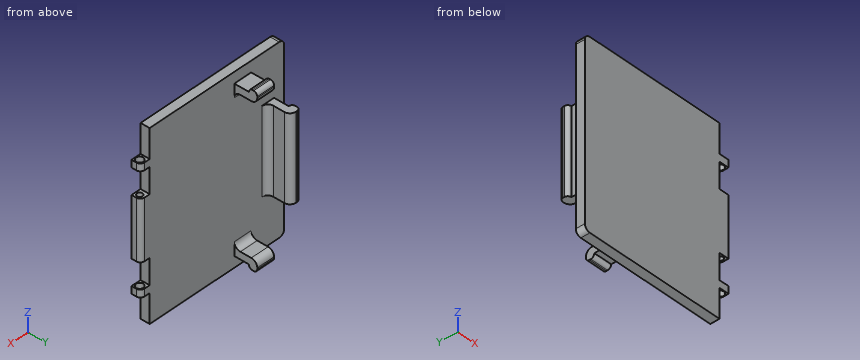
from build123d import *

# Parameters (mm, degrees)
EXTRUDE_START       = 0.25
EXTRUDE_BASE_DEPTH  = 3.75
FILLET1_R           = 1.75
SKETCH2_W           = 4
SKETCH2_H           = 10.5
SKETCH2_H_2         = 11.8971
CUT_EXTRUDE2_DEPTH  = 70.879033956
SKETCH4_R           = 1.5
CUT_EXTRUDE3_DEPTH  = 87.315736962
SKETCH6_W           = 3
SKETCH6_H           = 17.5
SKETCH6_W_2         = 7.5
SKETCH6_H_2         = 3
BOSS_EXTRUDE2_DEPTH = 9.5
SKETCH7_W           = 1.5
SKETCH7_H           = 3.5
BOSS_EXTRUDE3_DEPTH = 35
SKETCH8_W           = 1.5
SKETCH8_H           = 3.5
BOSS_EXTRUDE4_DEPTH = 7.5
SKETCH9_W           = 1.5
SKETCH9_H           = 3.5
BOSS_EXTRUDE5_DEPTH = 7.5
FILLET2_R           = 1.5
FILLET3_R           = 2.5
BOSS_EXTRUDE6_START = -24.5
SKETCH11_R          = 1.5
SKETCH11_R_2        = 1.125
BOSS_EXTRUDE6_DEPTH = 24.5


# Some blends are built 0.0001 mm under size
with BuildPart() as part:
    # Sketch1 → Extrude Base (new body)
    with BuildSketch(Plane.XZ.offset(10.085054916).offset(EXTRUDE_START)):
        with BuildLine():
            Line((56.857940404, 38.199863775), (56.857940404, -32.594336225))
            ThreePointArc((56.857940404, -32.594336225), (56.198930662, -34.185326483), (54.607940404, -34.844336225))
            Line((54.607940404, -34.844336225), (-4.892059596, -34.844336225))
            ThreePointArc((-4.892059596, -34.844336225), (-6.483049854, -34.185326483), (-7.142059596, -32.594336225))
            Line((-7.142059596, -32.594336225), (-7.142059596, 38.199863775))
            ThreePointArc((-7.142059596, 38.199863775), (-6.483049854, 39.790854032), (-4.892059596, 40.449863775))
            Line((-4.892059596, 40.449863775), (54.607940404, 40.449863775))
            ThreePointArc((54.607940404, 40.449863775), (56.198930662, 39.790854032), (56.857940404, 38.199863775))
        make_face()
    extrude(amount=EXTRUDE_BASE_DEPTH)

    # Fillet1
    # the kernel refuses this fillet: 1.75 mm, written as the material it takes off along each edge
    with BuildSketch(Plane(origin=(56.857940404, -10.335054916, 42.574863775), x_dir=(0, -1, 0), z_dir=(0, 0, -1))) as fillet1_piece_1:
        with BuildLine():
            CenterArc((FILLET1_R, FILLET1_R), FILLET1_R, 180, 90)
            Line((0, FILLET1_R), (0, 0))
            Line((0, 0), (FILLET1_R, 0))
        make_face()
    extrude(amount=79.5442, mode=Mode.SUBTRACT)

    # Sketch2 → Cut-Extrude2 (cut, through all)
    with BuildSketch(Plane.XZ.offset(14.085054916)):
        with Locations((54.857940404, 20.302763775)):
            Rectangle(SKETCH2_W, SKETCH2_H)
        with Locations((54.857940404, -14.697236225)):
            Rectangle(SKETCH2_W, SKETCH2_H)
        with Locations((54.857940404, -28.895786225)):
            Rectangle(SKETCH2_W, SKETCH2_H_2)
        with Locations((54.857940404, 34.501313775)):
            Rectangle(SKETCH2_W, SKETCH2_H_2)
    extrude(amount=-CUT_EXTRUDE2_DEPTH, mode=Mode.SUBTRACT)

    # Sketch4 → Cut-Extrude3 (cut, through all)
    with BuildSketch(Plane(origin=(0, 0, -22.947236225), x_dir=(-1, 0, 0), z_dir=(0, 0, -1))):
        with Locations(Location((-55.107940404, -12.335054916, 0), (0, 0, 90))):
            Circle(SKETCH4_R)
    extrude(amount=-CUT_EXTRUDE3_DEPTH, mode=Mode.SUBTRACT)

    # Sketch6 → Boss-Extrude2 (add)
    with BuildSketch(Plane(origin=(0, -10.335054916, 0), x_dir=(1, 0, 0), z_dir=(0, 1, 0))):
        with Locations((-1.142059596, -11.552763775)):
            Rectangle(SKETCH6_W, SKETCH6_H)
        with Locations((-1.142059596, 5.947236225)):
            Rectangle(SKETCH6_W, SKETCH6_H)
        with Locations((11.357940404, 28.844336225)):
            Rectangle(SKETCH6_W_2, SKETCH6_H_2)
        with Locations((11.357940404, -34.449863775)):
            Rectangle(SKETCH6_W_2, SKETCH6_H_2)
    extrude(amount=BOSS_EXTRUDE2_DEPTH)

    # Sketch7 → Boss-Extrude3 (add)
    with BuildSketch(Plane.XY.offset(20.302763775)):
        with Locations((-3.392059596, -2.585054916)):
            Rectangle(SKETCH7_W, SKETCH7_H)
    extrude(amount=-BOSS_EXTRUDE3_DEPTH)

    # Sketch8 → Boss-Extrude4 (add)
    with BuildSketch(Plane(origin=(15.107940404, 0, 0), x_dir=(0, 0, -1), z_dir=(1, 0, 0))):
        with Locations((31.094336225, -2.585054916)):
            Rectangle(SKETCH8_W, SKETCH8_H)
    extrude(amount=-BOSS_EXTRUDE4_DEPTH)

    # Sketch9 → Boss-Extrude5 (add)
    with BuildSketch(Plane(origin=(15.107940404, 0, 0), x_dir=(0, 0, -1), z_dir=(1, 0, 0))):
        with Locations((-36.699863775, -2.585054916)):
            Rectangle(SKETCH9_W, SKETCH9_H)
    extrude(amount=-BOSS_EXTRUDE5_DEPTH)

    # Fillet2
    fillet2_edges = [part.edges().sort_by_distance(p)[0] for p in [
        (11.357940404, -0.835054916, -31.844336225),
        (11.357940404, -4.335054916, -31.844336225),
        (-4.142059596, -0.835054916, 2.802763775),
        (-4.142059596, -4.335054916, 2.802763775),
        (11.357940404, -0.835054916, 37.449863775),
        (11.357940404, -4.335054916, 37.449863775),
    ]]
    fillet(fillet2_edges, radius=FILLET2_R - 0.0001)  # a hair under: the kernel refuses the full size

    # Fillet3
    fillet3_edges = [part.edges().sort_by_distance(p)[0] for p in [
        (0.357940404, -10.335054916, 2.802763775),
        (0.357940404, -0.835054916, 2.802763775),
        (11.357940404, -10.335054916, -27.344336225),
        (11.357940404, -0.835054916, -27.344336225),
        (11.357940404, -0.835054916, 32.949863775),
        (11.357940404, -10.335054916, 32.949863775),
    ]]
    fillet(fillet3_edges, radius=FILLET3_R)

    # Sketch11 → Boss-Extrude6 (add)
    with BuildSketch(Plane.XY.offset(15.052763775).offset(BOSS_EXTRUDE6_START)):
        with Locations(Location((55.107940404, -12.335054916, 0), (0, 0, 90))):
            Circle(SKETCH11_R)
        with Locations((55.107940404, -12.335054916)):
            Circle(SKETCH11_R_2, mode=Mode.SUBTRACT)
    extrude(amount=BOSS_EXTRUDE6_DEPTH)


solid = part.part
Work out the finished part from the listing and answer in its coordinate system (mm). Coordinates: 2 decimals unless noted, no trailing zeros. Write each loop counter-clockwise with the first axis right and the second up, starting at its lowest first coordinate (ties: lowest second). Pieces come first, ordered by that corner, then holes.
1. Flat-ended cylindrical pins translate along their axes: pin 1 (5 mm diameter, centred on y = -6, z = 8.5, fed in from +X); pin 2 (3.5 mm diameter, centred on x = 55.11, y = -12.34, fed in from -Z); pin 3 (4 mm diameter, centred on y = -11.5, z = -15, fed in from +X); pin 4 (4 mm diameter, centred on x = 54.5, y = -13, fed in from -Z). Find the tip coordinate at first contact, or state that the pin passes through.
Results list:
pin 1: stops at x = 0.45
pin 2: stops at z = -22.95
pin 3: stops at x = 52.86
pin 4: stops at z = -34.84
2. The part is cut by section C-C, the plane x = 49.5. Write down the section's boundary in (y, z).
Results list:
outline: (-14.09, -34.84) - (-10.34, -34.84) - (-10.34, 40.45) - (-14.09, 40.45) - close
3. Consider line 1 along X through (y, z) = (-12.5, -9); line 2 along Y through (x, z) = (30, 21.5); line 3 along X through (y, z) = (-6.25, -5). Determine where each line is inside the solid, lowest interval first.
Results list:
line 1: x = -7.14 to 54, 56.22 to 56.86
line 2: y = -14.09 to -10.34
line 3: x = -2.64 to 0.36
4. The part is cut by section D-D, the plane z = 31.5. Write down the section's boundary in (x, y), and give its area (3 significant figures).
Results list:
outline: (-7.14, -14.09) - (52.86, -14.09) - (52.86, -10.34) - (15.11, -10.34) - (15.11, -10.1) - (7.61, -10.1) - (7.61, -10.34) - (-7.14, -10.34) - close
area: 227 mm2
5. The part is cut by section A-A, the plane y = -6. Write down the section's boundary in (x, z).
Results list:
outline: (-2.64, -14.7) - (0.36, -14.7) - (0.36, 20.3) - (-2.64, 20.3) - close; (7.61, -30.34) - (15.11, -30.34) - (15.11, -27.34) - (7.61, -27.34) - close; (7.61, 32.95) - (15.11, 32.95) - (15.11, 35.95) - (7.61, 35.95) - close
